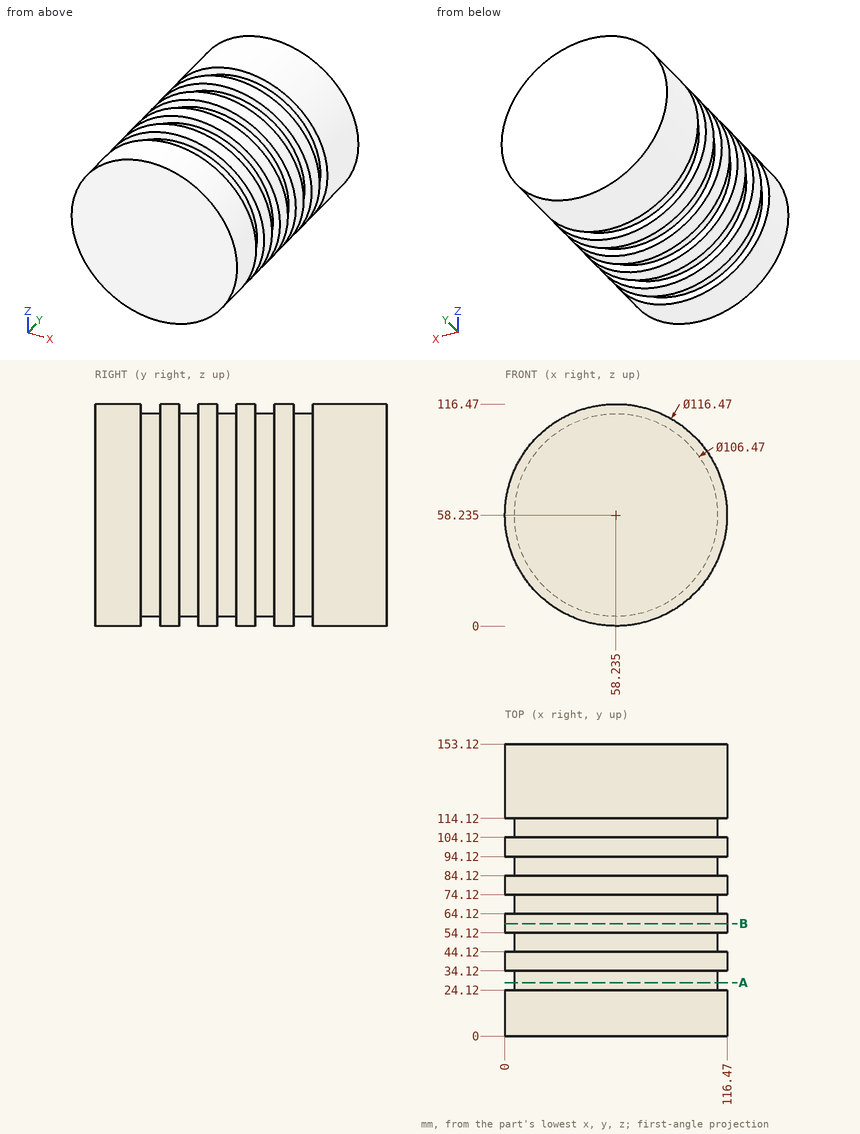
Source: three-view drawing plus pictorial views. Frame: mm from the lowest corner of the part. Give positions to 0.01 mm unless a question says otherwise; leave off trailing zeros. Order: outer loops, then holes, each group sorted by start corner. A loop starts at its lowest first (then second) coordinate and runs counter-clockwise, first axis right, second up. Notation, with made-up numbers: (88.25, -37.5) -> (132.25, -37.5) arc R25 ccw to (132.25, -22.5) -> close; hole circle Ø6 at (67, 7.25). An arc over 180 degrees is marked (long way). Use a Markdown table: item, result.
Q1. Section A-A (y = 28). Return the cut outline in (x, z) (3 decimals).
A:
| item | result |
|---|---|
| outline | circle Ø106.47 at (58.235, 58.235) |
Q2. Material intervals for line 1 (Z direction, x = 46, y = 8.5); line 2 (Z direction, x = 9, y = 65.5); line 3 (X direction, y = 56, z = 15.5), sorted ascending. Write a range as [from, to].
A:
| item | result |
|---|---|
| line 1 | [1.3, 115.17] |
| line 2 | [37.99, 78.48] |
| line 3 | [18.67, 97.8] |
Q3. Section B-B (y = 59). Return the cut outline in (x, z) (3 decimals), and give its area (3 significant figures).
A:
| item | result |
|---|---|
| outline | circle Ø116.47 at (58.235, 58.235) |
| area | 10,700 mm^2 |
Q4. First-contact query: P1, Ø6, axis at y = 37, z = 102.5, coming from the +X side; P2, Ø1, axis at x = 17.5, y = 104.5, coming from the -Z side; P3, Ø1, axis at x = 74, z = 25, coming from the -Y side; P4, Ø2, axis at x = 98, y = 38.5, coming from the +Z side. Flat tips, straight axial feed; report the tip coordinate or a pass-through.
A:
| item | result |
|---|---|
| P1 | x = 99.33 |
| P2 | z = 16.3 |
| P3 | y = 0 |
| P4 | z = 101.69 |
